Autodesk Inventor part; units mm, degrees
ref_plane "YZ Plane" through (0, 0, 0) normal (1, 0, 0) x (0, 1, 0)
ref_plane "XZ Plane" through (0, 0, 0) normal (0, 1, 0) x (-1, 0, 0)
ref_plane "XY Plane" through (0, 0, 0) normal (0, 0, 1) x (1, 0, 0)
ref_plane "Work Plane1" through (0, 0, 0) normal (0, 0, 1) x (1, 0, 0)
sketch "Sketch1" plane through (0, 0, 0) normal (0, 0, 1) x (1, 0, 0)
  line L0 (91, 0.01) -> (-91, 0.01) construction
  line L1 (91, 0.01) -> (91, 13.01) construction
  line L2 (28.25, 66.26) -> (91, 13.01) construction
  line L3 (-75.75, 66.26) -> (28.25, 66.26) construction
  line L4 (-91, 51.01) -> (-75.75, 66.26) construction
  line L5 (-91, 0.01) -> (-91, 51.01) construction
  circle A0 centre (22, 59.26) radius 1.95
  circle A1 centre (-84, 6.26) radius 1.95
  circle A2 centre (-84, 45.26) radius 1.95
  circle A3 centre (-70, 59.26) radius 1.95
  line L6 (149.1, -0.3275) -> (149.1, 180.6725) construction
  line L7 (-91, 0.01) -> (149, 0.01)
  line L8 (149, 0.01) -> (149, 66.26)
  line L9 (149, 66.26) -> (-91, 66.26)
  line L10 (-91, 66.26) -> (-91, 0.01)
  circle A4 centre (84, 6.26) radius 1.95
  point P0 (0, 0)
  dimension "d0" = 0.1
extrude "Extrusion1" add sketch "Sketch1" along normal blind 5
sketch "Sketch2" plane through (0, 0, 5) normal (0, 0, 1) x (1, 0, 0)
  line L0 (149, 0.01) -> (149, 66.26)
  line L1 (149, 66.26) -> (-91, 66.26)
  line L2 (149, 0.01) -> (144, 0.01)
  line L3 (144, 0.01) -> (144, 66.26)
  line L4 (144, 66.26) -> (149, 66.26)
  line L5 (149, 66.26) -> (149, 0.01)
  point P0 (0, 0)
  dimension "d3" = 5
extrude "Extrusion2" add sketch "Sketch2" along normal blind 20
fillet "Fillet1" radius 5 1 edges at (144, 33.135, 5)
sketch "Sketch3" plane through (-91, 66.26, 0) normal (0, 1, 0) x (1, 0, 0)
  line L0 (240, -25) -> (235, -25)
  line L1 (235, -25) -> (210, -5)
  line L2 (230, -5) -> (0, -5)
  line L3 (235, -10) -> (235, -25)
  arc A0 (235, -10) -> (230, -5) centre (230, -10) ccw
  point P0 (91, 0)
  dimension "d7" = 20
extrude "Extrusion3" add sketch "Sketch3" against normal blind 5
ref_plane "Work Plane2" through (-91, 33.135, 0) normal (0, -1, 0) x (1, 0, 0)
mirror "Mirror1" about plane through (-91, 33.135, 0) normal (0, -1, 0) of "Extrusion3"
sketch "Sketch4" plane through (144, 61.26, 10) normal (-1, 0, 0) x (0, 0, 1)
  line L0 (0, -56.25) -> (15, -56.25)
  line L1 (15, 0) -> (15, -56.25)
  line L2 (15, 0) -> (0, 0)
  line L3 (0, -56.25) -> (0, 0)
  circle A0 centre (7.5, -18.125) radius 2.5
  circle A1 centre (7.5, -38.125) radius 2.5
  circle A2 centre (7.5, -28.125) radius 2.5
  line L4 (0, -56.25) -> (0, 0)
  line L5 (0, -28.125) -> (15, -28.125) construction
  line L6 (15, -61.25) -> (15, 5)
  circle A3 centre (7.5, -8.125) radius 2.5
  circle A4 centre (7.5, -48.125) radius 2.5
  point P0 (-10, -61.26)
  point P1 (7.5, -28.125)
  dimension "d10" = 5
  dimension "d11" = 5
  dimension "d12" = 10
  dimension "d13" = 5
  dimension "d14" = 10
extrude "Extrusion4" cut sketch "Sketch4" against normal through all contours A0 | A1 | A2 | A3 | A4
properties part number "dilution system bracket"
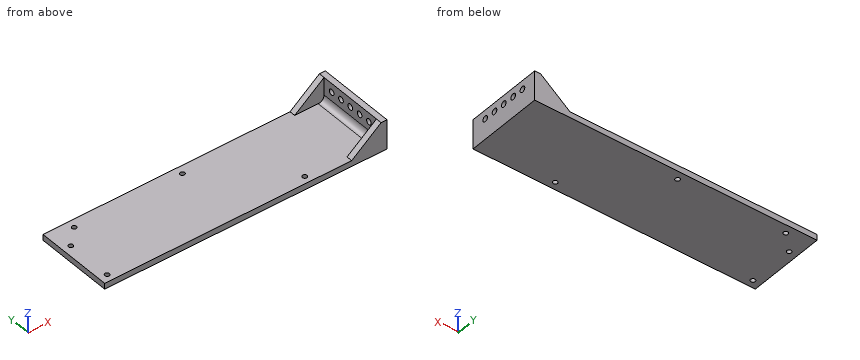
CAD build for the part. Positions are in the model's coordinates, mm. Round coordinates to 2 decimals unless told otherwise and drop trailing zeros. Loops run counter-clockwise (first coordinate to the right, second up) from the corner with the lowest first, then second, coordinate; pieces in that order, holes last. Notation, with made-up numbers: M 39.5,38.5 L 57.5,38.5 A9 cw 57.5,55.5 Z; hole C 86.25,36.5 d6. An arc over 180 degrees is marked long. Use a Markdown table: item, result. Add a question column.
(1) Flat gauge pins, fed straight in: pin 1 (1 mm diameter, centred on x = 60.5, y = 16, fed in from +Z); pin 2 (5 mm diameter, centred on y = 15, z = 8.5, fed in from -X); pin 3 (8 mm diameter, centred on y = 53.135, z = 17.5, fed in from -X). Where does each tip first touch, or does it go through?
(2) Cut at B-B (x = -25.5). Give the cut face in (y, z).
(3) Drill centre lines: line 1 (Y direction, x = 147.9, z = 17.5) (3 decimals); line 2 (Y direction, x = -84, z = 3.65); line 3 (X direction, y = 35, z = 19.5). Where is each one in solid material? Low to high.
(4) Cut at A-A (z = 17.5). Give the cut face in (x, y) (3 decimals), and give its area (3 significant figures).
Geometry says:
| question | item | result |
|---|---|---|
| 1 | pin 1 | stops at z = 5 |
| 1 | pin 2 | stops at x = 142 |
| 1 | pin 3 | stops at x = 144 |
| 2 | outline | M 0.01,0 L 66.26,0 L 66.26,5 L 0.01,5 Z |
| 3 | line 1 | y = 0.01 to 10.635, 15.635 to 20.635, 25.635 to 30.635, 35.635 to 40.635, 45.635 to 50.635, 55.635 to 66.26 |
| 3 | line 2 | y = 0.01 to 4.31, 8.21 to 43.31, 47.21 to 66.26 |
| 3 | line 3 | x = 144 to 149 |
| 4 | outline | M 134.625,0.01 L 149,0.01 L 149,10.635 L 144,10.635 L 144,5.01 L 134.625,5.01 Z; M 134.625,61.26 L 144,61.26 L 144,55.635 L 149,55.635 L 149,66.26 L 134.625,66.26 Z; M 144,15.635 L 149,15.635 L 149,20.635 L 144,20.635 Z; M 144,25.635 L 149,25.635 L 149,30.635 L 144,30.635 Z; M 144,35.635 L 149,35.635 L 149,40.635 L 144,40.635 Z; M 144,45.635 L 149,45.635 L 149,50.635 L 144,50.635 Z |
| 4 | area | 300 mm² |
